Geometry check sheet. Reference: the model listing, model coordinates, mm. A direction names the side the tool comes from. Coordinates: 2 decimals unless noted, no trailing zeros. Write each loop counter-clockwise with the first axis right and the second up, starting at its lowest first coordinate (ties: lowest second). Pieces come first, ordered by that corner, then holes.
from build123d import *

# Parameters (mm, degrees)
BOSS_EXTRUDE1_DEPTH  = 112
SKETCH2_R            = 3.025
CUT_EXTRUDE1_DEPTH   = 8
SKETCH3_W            = 11
SKETCH3_H            = 11
BOSS_EXTRUDE2_DEPTH  = 3.175
FILLET1_R            = 2
M4_CLEARANCE_HOLE1_D = 4.5


with BuildPart() as part:
    # Sketch1 → Boss-Extrude1 (new body)
    with BuildSketch(Plane.XY):
        with BuildLine():
            ThreePointArc((0, -13), (-9.192388155, -9.192388155), (-13, 0))
            Line((-13, 0), (-20.724457785, 0))
            Line((-20.724457785, 0), (-20.724457785, -13))
            Line((-20.724457785, -13), (0, -13))
        make_face()
        with BuildLine():
            Line((-11, 0), (-13, 0))
            ThreePointArc((-13, 0), (-9.192388155, -9.192388155), (0, -13))
            ThreePointArc((0, -13), (9.192388155, -9.192388155), (13, 0))
            Line((13, 0), (11, 0))
            ThreePointArc((11, 0), (0, -11), (-11, 0))
        make_face()
    extrude(amount=BOSS_EXTRUDE1_DEPTH)

    # Sketch2 → Cut-Extrude1 (cut)
    with BuildSketch(Plane(origin=(0, 0, 0), x_dir=(1, 0, 0), z_dir=(0, 1, 0))):
        with Locations(Location((-15.862228893, -25.4, 0), (0, 0, 180))):
            Circle(SKETCH2_R)
        with Locations(Location((-15.862228893, -86.6, 0), (0, 0, 180))):
            Circle(SKETCH2_R)
    extrude(amount=-CUT_EXTRUDE1_DEPTH, mode=Mode.SUBTRACT)

    # Sketch3 → Boss-Extrude2 (add)
    with BuildSketch(Plane.XZ.offset(13)):
        with Locations((-15.224457785, 117.5)):
            Rectangle(SKETCH3_W, SKETCH3_H)
        with Locations((-15.224457785, -5.5)):
            Rectangle(SKETCH3_W, SKETCH3_H)
    extrude(amount=-BOSS_EXTRUDE2_DEPTH)

    # Fillet1
    fillet1_edges = [part.edges().sort_by_distance(p)[0] for p in [
        (-20.724457785, -11.4125, 123),
        (-9.724457785, -11.4125, 123),
        (-20.724457785, -11.4125, -11),
        (-9.724457785, -11.4125, -11),
    ]]
    fillet(fillet1_edges, radius=FILLET1_R)

    # M4 Clearance Hole1 (through all)
    with Locations(Plane(origin=(0, -13, 0), x_dir=(-1, 0, 0), z_dir=(0, -1, 0))):
        with Locations((15.224457785, 5.5), (15.224457785, -117.5)):
            Hole(M4_CLEARANCE_HOLE1_D / 2)


solid = part.part
1. Sectioned sample at B-B, the plane y = -1.75. Record the boundary of the cut face in (x, z) (3 decimals), and give its area (3 significant figures).
Computed values:
outline: (-20.724, 0) - (-10.86, 0) - (-10.86, 112) - (-20.724, 112) - close; (10.86, 0) - (12.882, 0) - (12.882, 112) - (10.86, 112) - close; hole circle Ø6.05 at (-15.862, 25.4); hole circle Ø6.05 at (-15.862, 86.6)
area: 1,270 mm2
2. Sectioned sample at A-A, the plane z = 117.5. Record the boundary of the cut face in (x, y) (3 decimals), and give its area (3 significant figures).
Computed values:
outline: (-20.724, -13) - (-17.474, -13) - (-17.474, -9.825) - (-20.724, -9.825) - close; (-12.974, -13) - (-9.724, -13) - (-9.724, -9.825) - (-12.974, -9.825) - close
area: 20.6 mm2
3. Gauge pin test, flat ends, axial feed: pin 1 Ø2 at (x, z) = (4.5, 6.5) entering from +Y; pin 2 Ø3 at (x, z) = (5, 104.5) entering from -Y; pin 3 Ø1.6 at (y, z) = (-11.5, 116) entering from +X; pin 4 Ø5 at (x, z) = (-16.5, 26.5) entering from +Y. Record the tip position at first contact, or that the pin passes through.
Computed values:
pin 1: stops at y = -9.53
pin 2: stops at y = -12.52
pin 3: stops at x = -9.72
pin 4: stops at y = 0
4. Draft check along X on faces 1 (the cylindrical face through (-17.258, -3.944, 83.916)), 2 (the flat face through (-15, -11, 123)), 3 (the cylindrical face through (-17.472, -11.39, -5.599)), 4 (the cylindrical face through (9.091, -9.293, 55.216)). Enter one of: released by +X, released by -X, zero draft, split by the parting line, or undercut.
Computed values:
face 1: undercut
face 2: zero draft
face 3: undercut
face 4: released by +X
5. Thickness scan on line 1 along X through (y, z) = (-11.4, 117.5); line 2 along Z through (x, y) = (-13.5, -7.5); line 3 along X through (y, z) = (-2.75, 87). Record the ranges inside material, lowest first.
Computed values:
line 1: x = -20.72 to -17.47, -12.97 to -9.72
line 2: z = 0 to 23.51, 27.29 to 84.71, 88.49 to 112
line 3: x = -20.72 to -18.86, -12.86 to -10.65, 10.65 to 12.71
6. Sectioned sample at C-C, the plane z = 86.6. Record the boundary of the cut face in (x, y).
Computed values:
outline: (-20.72, -13) - (0, -13) arc R13 ccw to (13, 0) - (11, 0) arc R11 cw to (-11, 0) - (-12.84, 0) - (-12.84, -8) - (-18.89, -8) - (-18.89, 0) - (-20.72, 0) - close
7. Access from +Z, -Z, +X, -X, +Y, -Y to the whole of each face (thin tool, end or side, straight path). Record for faces 5 (the flat face through (-16, -8, 25)), 6 (the flat face through (-9.724, -11, 116)), 7 (the flat face through (-9.724, -11, -5)), 8 (the flat face through (-15, -9.825, -3)).
Computed values:
face 5: +Y
face 6: +Z, +X, +Y, -Y
face 7: -Z, +X, +Y, -Y
face 8: -Z, +X, -X, +Y
8. Sectioned sample at D-D, the plane x = -14.5. Record the boundary of the cut face in (y, z) (3 decimals), and give its area (3 significant figures).
Computed values:
outline: (-13, -11) - (-9.825, -11) - (-9.825, -7.63) - (-13, -7.63) - close; (-13, -3.37) - (-9.825, -3.37) - (-9.825, 0) - (0, 0) - (0, 22.699) - (-8, 22.699) - (-8, 28.101) - (0, 28.101) - (0, 83.899) - (-8, 83.899) - (-8, 89.301) - (0, 89.301) - (0, 112) - (-9.825, 112) - (-9.825, 115.37) - (-13, 115.37) - close; (-13, 119.63) - (-9.825, 119.63) - (-9.825, 123) - (-13, 123) - close
area: 1,410 mm2
